```python
from build123d import *

# Parameters (mm, degrees)
SKETCH1_R           = 50.4825
BOSS_EXTRUDE1_DEPTH = 2.5908
SKETCH2_R           = 47.4472
BOSS_EXTRUDE2_DEPTH = 4.6482
SKETCH3_R           = 3.2
SKETCH3_R_2         = 3.22
SKETCH3_R_3         = 3.302
CUT_EXTRUDE1_DEPTH  = 8.239


with BuildPart() as part:
    # Sketch1 → Boss-Extrude1 (new body)
    with BuildSketch(Plane(origin=(0, 0, 0), x_dir=(1, 0, 0), z_dir=(0, 1, 0))):
        Circle(SKETCH1_R)
    extrude(amount=BOSS_EXTRUDE1_DEPTH)

    # Sketch2 → Boss-Extrude2 (add)
    with BuildSketch(Plane(origin=(0, 2.5908, 0), x_dir=(1, 0, 0), z_dir=(0, 1, 0))):
        Circle(SKETCH2_R)
    extrude(amount=BOSS_EXTRUDE2_DEPTH)

    # Sketch3 → Cut-Extrude1 (cut, through all)
    with BuildSketch(Plane.XZ):
        with Locations((-38.852, 0)):
            Circle(SKETCH3_R)
        with Locations((38.85200002, 0)):
            Circle(SKETCH3_R_2)
        Circle(SKETCH3_R_3)
    extrude(amount=-CUT_EXTRUDE1_DEPTH, mode=Mode.SUBTRACT)


solid = part.part
```
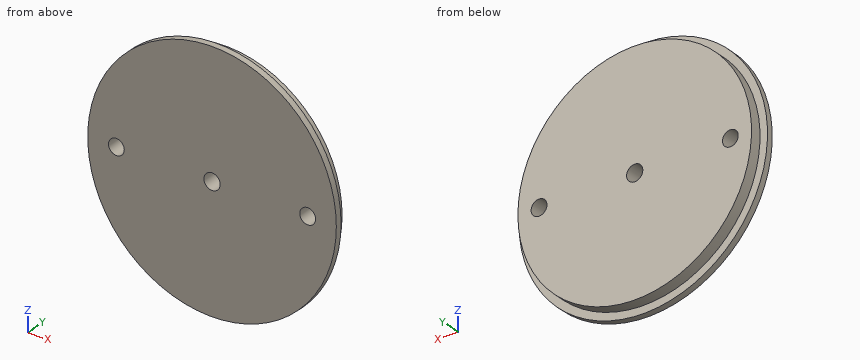
Can you work these out from the model? Positions are in its coordinate system, mm. Round coordinates to 2 decimals unless told otherwise and drop trailing zeros. Loops run counter-clockwise (first coordinate to the right, second up) from the corner with the lowest first, then second, coordinate; pieces in that order, holes last.
Item 1: Suppose I cut it at A-A, the plane x = 0. Write out the boundary of the cut face in (y, z), then the cut area to 3 significant figures.
Item 2: Suppose I cut it at D-D, the plane y = 1.25. Write out the boundary of the cut face in (x, z) (1 decimal), then the cut area to 3 significant figures.
Item 3: Suppose I cut it at B-B, the plane z = 0. Write out the boundary of the cut face in (x, y), then the cut area to 3 significant figures.
Item 4: Suppose I cut it at C-C, the plane z = -19.5. Write out the boundary of the cut face in (x, y).
Item 5: Please list where these lines run through material, in increasing order: L1, parallel to Z at x = -1.5, y = 7; L2, parallel to Z at x = 35, y = 7; L3, parallel to Z at x = 43, y = 6.
Item 6: Will these pins go through, and if not, where does the flat tip stop? pin 1 Ø10 at (x, z) = (15.5, 35) entering from -Y; pin 2 Ø2 at (y, z) = (3.5, -23) entering from +X; pin 3 Ø2 at (y, z) = (5, -17.5) entering from +X.
Reported:
1. outline: (0, -50.48) - (2.59, -50.48) - (2.59, -47.45) - (7.24, -47.45) - (7.24, -3.3) - (0, -3.3) - close; (0, 3.3) - (7.24, 3.3) - (7.24, 47.45) - (2.59, 47.45) - (2.59, 50.48) - (0, 50.48) - close
1. area: 655 mm2
2. outline: circle Ø101 at (0, 0); hole circle Ø6.4 at (-38.9, 0); hole circle Ø6.6 at (0, 0); hole circle Ø6.4 at (38.9, 0)
2. area: 7,910 mm2
3. outline: (-50.48, 0) - (-42.05, 0) - (-42.05, 7.24) - (-47.45, 7.24) - (-47.45, 2.59) - (-50.48, 2.59) - close; (-35.65, 0) - (-3.3, 0) - (-3.3, 7.24) - (-35.65, 7.24) - close; (3.3, 0) - (35.63, 0) - (35.63, 7.24) - (3.3, 7.24) - close; (42.07, 0) - (50.48, 0) - (50.48, 2.59) - (47.45, 2.59) - (47.45, 7.24) - (42.07, 7.24) - close
3. area: 562 mm2
4. outline: (-46.56, 0) - (46.56, 0) - (46.56, 2.59) - (43.25, 2.59) - (43.25, 7.24) - (-43.25, 7.24) - (-43.25, 2.59) - (-46.56, 2.59) - close
5. L1: z = -47.42 to -2.94, 2.94 to 47.42
5. L2: z = -32.03 to 32.03
5. L3: z = -20.06 to 20.06
6. pin 1: stops at y = 0
6. pin 2: stops at x = 45.15
6. pin 3: stops at x = 44.49
